from build123d import *

# Parameters (mm, degrees)
F0_W     = 38.1
F0_H     = 25.4
F1_DEPTH = 25.4
F3_DEPTH = 25.4
F5_DEPTH = 19.05
F7_DEPTH = 558.8
F8_W     = 19.05
F8_H     = 6.35
F9_DEPTH = 25.4


with BuildPart() as f1:
    # F0 (on Front) → F1 (new body)
    with BuildSketch(Plane.XZ):
        with Locations((19.05, 12.7)):
            Rectangle(F0_W, F0_H)
    extrude(amount=F1_DEPTH)

    # F2 (on face) → F3 (cut)
    with BuildSketch(Plane.XZ.offset(25.4)):
        Polygon((12.7, 25.4), (0, 25.4), (0, 12.7), align=None)
        Polygon((38.1, 12.7), (38.1, 25.4), (25.4, 25.4), align=None)
    extrude(amount=-F3_DEPTH, mode=Mode.SUBTRACT)

    # F4 (on face) → F5 (cut)
    with BuildSketch(Plane.XZ.offset(25.4)):
        Polygon((0, 0), (19.05, 19.05), (38.1, 0), (38.1, 12.7), (25.4, 25.4), (12.7, 25.4), (0, 12.7), align=None)
    extrude(amount=-F5_DEPTH, mode=Mode.SUBTRACT)

    # F6 (on Right) → F7 (cut)
    with BuildSketch(Plane.YZ):
        Polygon((-25.4, 19.05), (-25.4, 0), (-6.35, 19.05), align=None)
    extrude(amount=F7_DEPTH, mode=Mode.SUBTRACT)

    # F8 (on face) → F9 (cut)
    with BuildSketch(Plane(origin=(0, 0, 0), x_dir=(1, 0, 0), z_dir=(0, 0, -1))):
        with Locations((19.05, 22.225)):
            Rectangle(F8_W, F8_H)
    extrude(amount=-F9_DEPTH, mode=Mode.SUBTRACT)


solid = f1.part
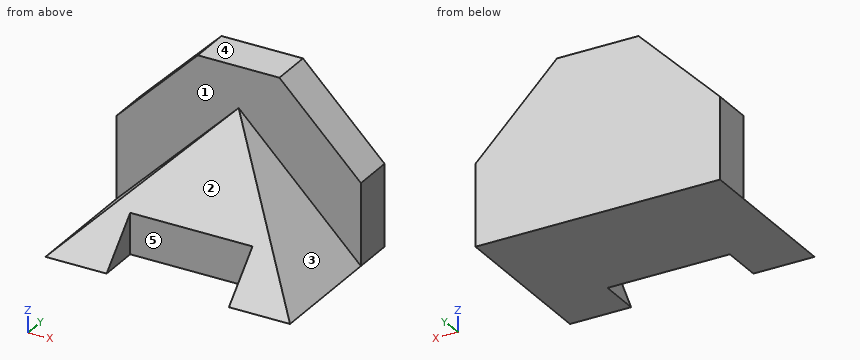
Can you work these out from the model? Positions are in its coordinate system, mm. Face numbers are marked on the shaded views. A direction names the side the tool comes from. Coordinates: 2 decimals unless noted, no trailing zeros. Order: outer loops, then holes, each group sorted by start corner. A loop starts at its lowest first (then second) coordinate and runs counter-clockwise, first axis right, second up. Notation, with made-up numbers: M 66.25,4 L 91.25,4 A12 ccw 91.25,21 Z; hole C 58.5,16 d3. An arc over 180 degrees is marked long. Answer as CSV lines item,"result".
(1) Suppose I cut it at B-B on z = 7.5. Please give me the cut outline in (x, y).
Geometry check:
outline,"M 0,-6.35 L 7.5,-6.35 L 7.5,-17.9 L 30.6,-17.9 L 30.6,-6.35 L 38.1,-6.35 L 38.1,0 L 0,0 Z"
(2) Suppose I cut it at D-D on x = 27.5. Please give me the cut outline in (y, z), plus the area to 3 significant figures.
Geometry check:
outline,"M -19.05,0 L 0,0 L 0,23.3 L -6.35,23.3 L -6.35,10.6 L -14.8,10.6 L -19.05,6.35 Z"
area,"274 mm^2"
(3) Suppose I cut it at C-C on y = -11.5. Please give me the cut outline in (x, z), plus the area to 3 significant figures.
Geometry check:
outline,"M 0,0 L 38.1,0 L 24.2,13.9 L 13.9,13.9 Z"
area,"336 mm^2"
(4) On a 3-axis mill with a long thin cutter (end or side, diameter ignored), from which of +Z, -Z, +X, -X, +Y, -Y can I reach the whole of each face in a straight line? I mean the marked faces 1 and 2. Say none if no direction works.
Geometry check:
face 1,"+Z, -Y"
face 2,"+Z, +X, -X, -Y"
(5) Please list where these lines run through material, in increasing order: L1, parallel to Y at x = 28.5, z = 21.25; L2, parallel to Y at x = 8.5, z = 2.5; L3, parallel to Z at x = 5.5, y = -20.5.
Geometry check:
L1,"-6.35 to 0"
L2,"-22.9 to 0"
L3,"0 to 4.9"
(6) I'm going to push flat-ended pins straight in: pin 1 (5 mm diameter, centred on x = 19, z = 19.5, fed in from +Y); pin 2 (10 mm diameter, centred on x = 32.5, y = -5.5, fed in from +Z); pin 3 (7 mm diameter, centred on y = -23.5, z = 4.5, fed in from +X); pin 4 (12 mm diameter, centred on y = -22.5, z = 7.5, fed in from +X). Where does each tip first touch, or does it pass through?
Geometry check:
pin 1,"y = 0"
pin 2,"z = 23.3"
pin 3,"x = 37.1"
pin 4,"x = 36.6"
(7) Suppose I cut it at A-A on x = 22. Please give me the cut outline in (y, z), plus the area to 3 significant figures.
Geometry check:
outline,"M -19.05,0 L 0,0 L 0,25.4 L -6.35,25.4 L -6.35,16.1 L -9.3,16.1 L -19.05,6.35 Z"
area,"318 mm^2"
(8) If we mould it in two halves opening along X, with no side actions, what happens to the marked faces 3, 4 and 5? For each: released by +X, released by -X, zero draft, split by the parting line, or undercut.
Geometry check:
face 3,"released by +X"
face 4,"zero draft"
face 5,"undercut"
